Source: CAD feature listing. Evaluate the final solid. Frame: model axes, mm. Give positions to 0.01 mm unless a question says otherwise; leave off trailing zeros. Loops run counter-clockwise (first coordinate to the right, second up) from the corner with the lowest first, then second, coordinate; pieces in that order, holes last.
```python
from build123d import *

# Parameters (mm, degrees)
F0_R     = 115
F1_DEPTH = 1.5


with BuildPart() as f1:
    # F0 (on Top) → F1 (new body, symmetric)
    with BuildSketch(Plane.XY):
        Polygon((-59.9971862603, -140.6090075683), (-55.7561938299, -144.85), (-29.9988345097, -144.85), (-29.9988345097, -141.85), (0, -141.85), (0, -144.85), (30, -144.85), (30, -141.85), (56.9988345097, -141.85), (62.9988345097, -141.85), (81.2120379453, -123.6367965644), (79.0907176018, -121.5154762208), (100.3039210374, -100.3022727852), (102.4252413809, -102.4235931288), (123.6384448165, -81.2103896932), (121.517124473, -79.0890693497), (140.609007565, -59.9971862576), (144.85, -55.7561938226), (144.85, -29.9988345097), (141.85, -29.9988345097), (141.85, 0.0011654903), (144.85, 0), (144.85, 30), (141.85, 30), (141.85, 57), (141.85, 62.9988345097), (123.6367965644, 81.2120379453), (121.5154762208, 79.0907176018), (100.3022727852, 100.3039210374), (102.4235931255, 102.4252413776), (81.2103896932, 123.6384448165), (79.0890693497, 121.517124473), (59.9971862576, 140.609007565), (55.7561938226, 144.85), (29.9988345097, 144.85), (29.9988345097, 141.85), (-0.0011654903, 141.85), (0, 144.85), (-30, 144.85), (-30, 141.85), (-57, 141.85), (-62.9988345097, 141.85), (-81.2120379453, 123.6367965644), (-79.0907176018, 121.5154762208), (-100.3039210374, 100.3022727852), (-102.4252413776, 102.4235931255), (-123.6384448165, 81.2103896932), (-121.5171244733, 79.0890693493), (-140.6090075683, 59.9971862603), (-144.85, 55.7561938286), (-144.85, 29.9988345097), (-141.85, 29.9988345097), (-141.85, -0.0011654903), (-144.85, 0), (-144.85, -30), (-141.85, -30), (-141.85, -57), (-141.85, -62.9988345097), (-123.6367965644, -81.2120379453), (-121.5154762208, -79.0907176018), (-100.3022727852, -100.3039210374), (-102.4235931255, -102.4252413776), (-81.2103896932, -123.6384448165), (-79.0890693493, -121.5171244733), align=None)
        Circle(F0_R, mode=Mode.SUBTRACT)
    extrude(amount=F1_DEPTH, both=True)


solid = f1.part
```
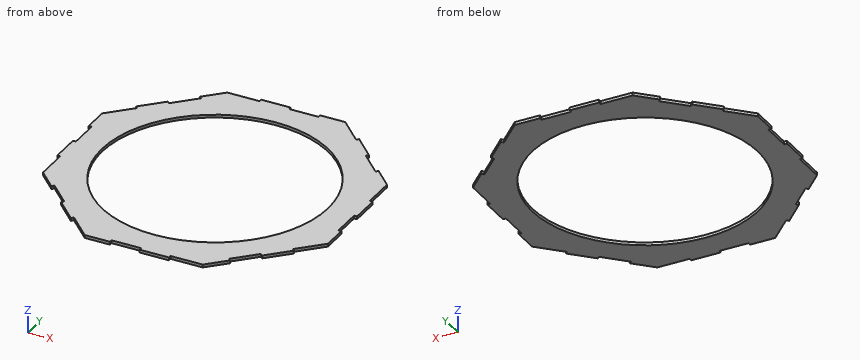
(1) Section A-A, the plane x = 96.5. Return the cut outline in (y, z).
A:
outline: (-104.11, -1.5) - (-62.55, -1.5) - (-62.55, 1.5) - (-104.11, 1.5) - close; (62.55, -1.5) - (108.35, -1.5) - (108.35, 1.5) - (62.55, 1.5) - close
(2) First-contact query: pin 1 (1.5 mm diameter, centred on x = -49.5, z = 0, fed in from +Y); pin 2 (0.9 mm diameter, centred on y = 14.5, z = -0.5, fed in from -X); pin 3 (1.5 mm diameter, centred on x = 45.5, z = 0, fed in from -Y). Flat tips, straight axial feed; report the tip coordinate or a pass-through.
A:
pin 1: stops at y = 141.85
pin 2: stops at x = -141.85
pin 3: stops at y = -141.85
(3) Section B-B, the plane y = -21. Return the cut outline in (x, z).
A:
outline: (-144.85, -1.5) - (-113.07, -1.5) - (-113.07, 1.5) - (-144.85, 1.5) - close; (113.07, -1.5) - (141.85, -1.5) - (141.85, 1.5) - (113.07, 1.5) - close
(4) Ray query, line 1 along X through (y, z) = (-24, 0); line 2 along X through (y, z) = (42, 1.3); line 3 along Y through (x, z) = (-103.5, -0.5). Return the intervals inside material, ascending.
A:
line 1: x = -144.85 to -112.47, 112.47 to 141.85
line 2: x = -144.85 to -107.06, 107.06 to 141.85
line 3: y = -97.11 to -50.13, 50.13 to 101.35
